from build123d import *

# Parameters (mm, degrees)
SCHIZZO1_R                   = 2.05
SCHIZZO1_W                   = 25
SCHIZZO1_H                   = 5
ESTRUSIONE_ESTRUSIONE2_DEPTH = 5
CUT_EXTRUDE1_REACH           = 7
SKETCH1_R                    = 2.05


with BuildPart() as part:
    # Schizzo1 → Estrusione-Estrusione2 (new body)
    with BuildSketch(Plane.XY):
        with BuildLine():
            Line((-22.627416998, -7.5), (0, -7.5))
            ThreePointArc((0, -7.5), (6.929096494, -2.870125743), (5.303300859, 5.303300859))
            Line((5.303300859, 5.303300859), (-17.324116139, 27.930717857))
            ThreePointArc((-17.324116139, 27.930717857), (-23.686333927, 30.052287026), (-29.20181593, 26.236749163))
            Line((-29.20181593, 26.236749163), (-45.934294533, 4.586300077))
            ThreePointArc((-45.934294533, 4.586300077), (-46.732282324, -3.305506726), (-40, -7.5))
            Line((-40, -7.5), (-22.627416998, -7.5))
        make_face()
        Circle(SCHIZZO1_R, mode=Mode.SUBTRACT)
        with Locations((-22.627416998, 22.627416998)):
            Circle(SCHIZZO1_R, mode=Mode.SUBTRACT)
        with Locations((-40, 0)):
            Circle(SCHIZZO1_R, mode=Mode.SUBTRACT)
        with Locations((-22.5, -2)):
            Rectangle(SCHIZZO1_W, SCHIZZO1_H, mode=Mode.SUBTRACT)
    extrude(amount=ESTRUSIONE_ESTRUSIONE2_DEPTH)

    # Sketch1 → Cut-Extrude1 (cut, up to next)
    with BuildSketch(Plane.XY.offset(5), mode=Mode.PRIVATE) as cut_extrude1_sk1:
        with Locations((-35, 0.5)):
            Circle(SKETCH1_R)
    cut_extrude1_tool1 = extrude(cut_extrude1_sk1.sketch, amount=-CUT_EXTRUDE1_REACH, mode=Mode.PRIVATE) & part.part
    add(cut_extrude1_tool1.solids().sort_by_distance((-35, 0.5, 5))[0], mode=Mode.SUBTRACT)
    # Sketch1 → Cut-Extrude1 (cut, up to next)
    with BuildSketch(Plane.XY.offset(5), mode=Mode.PRIVATE) as cut_extrude1_sk2:
        with Locations((-35, -4.5)):
            Circle(SKETCH1_R)
    cut_extrude1_tool2 = extrude(cut_extrude1_sk2.sketch, amount=-CUT_EXTRUDE1_REACH, mode=Mode.PRIVATE) & part.part
    add(cut_extrude1_tool2.solids().sort_by_distance((-35, -4.5, 5))[0], mode=Mode.SUBTRACT)
    # Sketch1 → Cut-Extrude1 (cut, up to next)
    with BuildSketch(Plane.XY.offset(5), mode=Mode.PRIVATE) as cut_extrude1_sk3:
        with Locations((-10, -4.5)):
            Circle(SKETCH1_R)
    cut_extrude1_tool3 = extrude(cut_extrude1_sk3.sketch, amount=-CUT_EXTRUDE1_REACH, mode=Mode.PRIVATE) & part.part
    add(cut_extrude1_tool3.solids().sort_by_distance((-10, -4.5, 5))[0], mode=Mode.SUBTRACT)
    # Sketch1 → Cut-Extrude1 (cut, up to next)
    with BuildSketch(Plane.XY.offset(5), mode=Mode.PRIVATE) as cut_extrude1_sk4:
        with Locations((-10, 0.5)):
            Circle(SKETCH1_R)
    cut_extrude1_tool4 = extrude(cut_extrude1_sk4.sketch, amount=-CUT_EXTRUDE1_REACH, mode=Mode.PRIVATE) & part.part
    add(cut_extrude1_tool4.solids().sort_by_distance((-10, 0.5, 5))[0], mode=Mode.SUBTRACT)


solid = part.part
Could you check a few things on this model? Use its own coordinates, in mm. A direction names the side the tool comes from. Coordinates: 2 decimals unless noted, no trailing zeros. Write each loop counter-clockwise with the first axis right and the second up, starting at its lowest first coordinate (ties: lowest second). Pieces come first, ordered by that corner, then holes. Notation, with made-up numbers: (68, 52) - (87, 52) arc R25 cw to (87, 87) - close; hole circle Ø10 at (43.5, 58). An arc over 180 degrees is marked (long way). Put each result on its own line as item: value. Start each with the question number.
Q1. I want a section at B-B on x = -15. Write out the boundary of the cut face in (y, z).
Q2. I want a section at D-D on y = 16. Write out the boundary of the cut face in (x, z), plus the area to 3 significant figures.
Q3. Thinking about a two-plate mould opening in Y: for faces 3 (the cylindrical face through (-8.5, 1.9, 2.5)), 4 (the flat face through (-20, -7.5, 2)), 5 (the flat face through (-5.852, 16.459, 2.465)), which applies, pulls with the +Y half, pulls with the -Y half, needs draft (parallel to the pull), parting line crosses it, or undercut?
Q4. I'm going to push flat-ended pins straight in: P1, Ø3.5, axis at x = -22.63, y = 22.63, coming from the -Z side; P2, Ø1.5, axis at y = 19, z = 0.5, coming from the +X side; P3, Ø2, axis at y = 4, z = 3.5, coming from the -X side; P4, Ø0.7, axis at y = -2, z = 3, coming from the +X side. Where does each tip first touch, or does it pass through?
Q5. I want a section at A-A on y = -3.5. Write out the boundary of the cut face in (x, z).
Q6. Which directions (+Z, -Z, +X, -X, +Y, -Y) give clear straight access to the entire face, cutting with the end or side of a thin tool? Please do faces 1 (the cylindrical face through (6.881, -2.984, 2.465)), 2 (the flat face through (-23, -4.5, 2)).
Q7. Please list where these lines run through material, in increasing order: L1, parallel to Y at x = -35.5, z = 1.55; L2, parallel to Y at x = -30.5, z = 0.65; L3, parallel to Y at x = 0, z = 2.6.
Q8. I want a section at C-C on z = 1.15. Write out the boundary of the cut face in (x, y), plus the area to 3 significant figures.
Checks:
1. outline: (-7.5, 0) - (-4.5, 0) - (-4.5, 5) - (-7.5, 5) - close; (0.5, 0) - (25.61, 0) - (25.61, 5) - (0.5, 5) - close
2. outline: (-37.11, 0) - (-5.39, 0) - (-5.39, 5) - (-37.11, 5) - close
2. area: 159 mm²
3. face 3: undercut
3. face 4: pulls with the -Y half
3. face 5: pulls with the +Y half
4. P1: through
4. P2: x = -7.64
4. P3: x = -46.87
4. P4: x = 7.32
5. outline: (-46.63, 0) - (-36.79, 0) - (-36.79, 5) - (-46.63, 5) - close; (-8.21, 0) - (6.63, 0) - (6.63, 5) - (-8.21, 5) - close
6. face 1: +Z, -Z, +X
6. face 2: +Z, -Z
7. L1: -7.5 to -6.49, -2.51 to -1.49, 2.49 to 18.09
7. L2: -7.5 to -4.5, 0.5 to 24.56
7. L3: -7.5 to -2.05, 2.05 to 10.61
8. outline: (-45.93, 4.59) arc R7.5 ccw to (-40, -7.5) - (0, -7.5) arc R7.5 ccw to (5.3, 5.3) - (-17.32, 27.93) arc R7.5 ccw to (-29.2, 26.24) - close; hole circle Ø4.1 at (-40, 0); hole (-35, -2.45) arc R2.05 ccw (long way) to (-32.95, -4.5) - (-12.05, -4.5) arc R2.05 ccw (long way) to (-10, -2.45) - (-10, -1.55) arc R2.05 ccw (long way) to (-12.05, 0.5) - (-32.95, 0.5) arc R2.05 ccw (long way) to (-35, -1.55) - close; hole circle Ø4.1 at (-22.63, 22.63); hole circle Ø4.1 at (0, 0)
8. area: 1,180 mm²
